```python
from build123d import *

# Parameters (mm, degrees)
SKETCH1_R           = 16.5
BOSS_EXTRUDE1_DEPTH = 26
CUT_EXTRUDE1_START  = -5
SKETCH2_R           = 16.5
SKETCH2_R_2         = 12.5
CUT_EXTRUDE1_DEPTH  = 5
SKETCH3_R           = 16.5
SKETCH3_R_2         = 15
CUT_EXTRUDE2_DEPTH  = 15
SKETCH4_R           = 12.5
CUT_EXTRUDE3_DEPTH  = 15


with BuildPart() as part:
    # Sketch1 → Boss-Extrude1 (new body)
    with BuildSketch(Plane(origin=(0, 0, 0), x_dir=(0, 1, 0), z_dir=(0, 0, 1))):
        with Locations(Location((0, 0, 0), (0, 0, 90))):
            Circle(SKETCH1_R)
    extrude(amount=BOSS_EXTRUDE1_DEPTH)

    # Sketch2 → Cut-Extrude1 (cut)
    with BuildSketch(Plane.XY.offset(26).offset(CUT_EXTRUDE1_START)):
        with Locations(Location((0, 0, 0), (0, 0, 180))):
            Circle(SKETCH2_R)
        Circle(SKETCH2_R_2, mode=Mode.SUBTRACT)
    extrude(amount=CUT_EXTRUDE1_DEPTH, mode=Mode.SUBTRACT)

    # Sketch3 → Cut-Extrude2 (cut)
    with BuildSketch(Plane(origin=(0, 0, 0), x_dir=(1, 0, 0), z_dir=(0, 0, -1))):
        with Locations(Location((0, 0, 0), (0, 0, 180))):
            Circle(SKETCH3_R)
        with Locations(Location((0, 0, 0), (0, 0, 180))):
            Circle(SKETCH3_R_2, mode=Mode.SUBTRACT)
    extrude(amount=-CUT_EXTRUDE2_DEPTH, mode=Mode.SUBTRACT)

    # Sketch4 → Cut-Extrude3 (cut)
    with BuildSketch(Plane(origin=(0, 0, 0), x_dir=(1, 0, 0), z_dir=(0, 0, -1))):
        Circle(SKETCH4_R)
    extrude(amount=-CUT_EXTRUDE3_DEPTH, mode=Mode.SUBTRACT)


solid = part.part
```
The listing builds one solid part. Answer for the finished solid, in the listing's coordinates (mm). A direction names the side the tool comes from. Round coordinates to 2 decimals unless told otherwise and drop trailing zeros. Loops run counter-clockwise (first coordinate to the right, second up) from the corner with the lowest first, then second, coordinate; pieces in that order, holes last.
1) For faces 4 (the face through (0, 0, 15)), 5 (the face through (12.3, -3.7, 21)), 6 (the face through (3.577, 16.108, 17.958)), determine the directions among +Z, -Z, +X, -X, +Y, -Y from which every point of the face is accessible in a straight line to the end or side of a thin tool.
Outcome:
face 4: -Z
face 5: +Z
face 6: +Z, -Z
2) Consider line 1 (Y direction, x = 0, z = 10.75); line 2 (Z direction, x = -2.5, y = 5); line 3 (Z direction, x = 10.5, y = -7). Determine where each line is inside the solid, lowest interval first.
Outcome:
line 1: y = -15 to -12.5, 12.5 to 15
line 2: z = 15 to 26
line 3: z = 0 to 21
3) A cutting plane is placed at D-D on z = 20. Determine the outline of the cut face in (x, y), plus the area to 3 significant figures.
Outcome:
outline: circle Ø33 at (0, 0)
area: 855 mm2
4) For a pull along X with two mould halves and no side action, classify faces 1 (the face through (11.923, 3.755, 23.465)), 2 (the face through (11.923, -3.755, 7.395)), 3 (the face through (3.4, -12.3, 0)) as released by +X, released by -X, zero draft, split by the parting line, or undercut.
Outcome:
face 1: split by the parting line
face 2: undercut
face 3: zero draft
5) A cutting plane is placed at B-B on z = 13.75. Determine the outline of the cut face in (x, y).
Outcome:
outline: circle Ø30 at (0, 0); hole circle Ø25 at (0, 0)
6) Given P1, Ø10, axis at x = 12, z = 9, coming from the +Y side; P2, Ø4, axis at x = -6.5, z = 6.5, coming from the +Y side; P3, Ø8, axis at y = 5, z = 14.5, coming from the -X side, each flat-ended and moving along its own axis, determine where each tip first touches the part or whether it passes through.
Outcome:
P1: stops at y = 13.27
P2: stops at y = 14.31
P3: stops at x = -16.47
7) A cutting plane is placed at A-A on x = 0. Determine the outline of the cut face in (y, z), plus the area to 3 significant figures.
Outcome:
outline: (-16.5, 15) - (-15, 15) - (-15, 0) - (-12.5, 0) - (-12.5, 15) - (12.5, 15) - (12.5, 0) - (15, 0) - (15, 15) - (16.5, 15) - (16.5, 21) - (12.5, 21) - (12.5, 26) - (-12.5, 26) - (-12.5, 21) - (-16.5, 21) - close
area: 398 mm2
